Design review of the part built by this model. Coordinates are the model's own, in mm. A direction names the side the tool comes from. Coordinates: 2 decimals unless noted, no trailing zeros. Order: outer loops, then holes, each group sorted by start corner. A loop starts at its lowest first (then second) coordinate and runs counter-clockwise, first axis right, second up. Notation, with made-up numbers: M 71.25,17.25 L 89.25,17.25 A20 ccw 89.25,36.25 Z; hole C 9,-24.5 d10. An arc over 180 degrees is marked long. Answer in a Markdown table with one row per item.
from build123d import *

# Parameters (mm, degrees)
PAD120_DEPTH    = 85
SKETCH241_R     = 1.5
POCKET086_DEPTH = 15.451
SKETCH242_W     = 25
SKETCH242_H     = 15.45
PAD121_DEPTH    = 4


with BuildPart() as part:
    # Sketch240 → Pad120 (new body)
    with BuildSketch(Plane.YZ):
        Polygon((-5.25, 11.45), (-5.25, 15.45), (19.75, 15.45), (19.75, 11.45), (11.25, 11.45), (11.25, 7.15), (14.5, 7.15), (14.5, 0), (0, 0), (0, 7.15), (3.25, 7.15), (3.25, 11.45), align=None)
    extrude(amount=PAD120_DEPTH)

    # Sketch241 (on Face2 of Pad120) → Pocket086 (cut, through all)
    with BuildSketch(Plane(origin=(0, 0, 15.45), x_dir=(0, -1, 0), z_dir=(0, 0, 1))):
        with Locations((-17.25, 77.5)):
            Circle(SKETCH241_R)
        with Locations((-17.25, 52.5)):
            Circle(SKETCH241_R)
        with Locations((2.75, 52.5)):
            Circle(SKETCH241_R)
        with Locations((2.75, 77.5)):
            Circle(SKETCH241_R)
    extrude(amount=-POCKET086_DEPTH, mode=Mode.SUBTRACT)

    # Sketch242 (on Face4 of Pocket086) → Pad121 (join)
    with BuildSketch(Plane(origin=(0, 0, 0), x_dir=(0, 1, 0), z_dir=(-1, 0, 0))):
        with Locations((7.25, -7.725)):
            Rectangle(SKETCH242_W, SKETCH242_H)
    extrude(amount=PAD121_DEPTH)


with BuildPart() as part_1:
    # Body140 placement: moved
    add(part.part.moved(Location((-115, 122.3, 7))))


solid = part_1.part
(1) For faces 4 (the flat face through (-73, 136.8, 11)), 5 (the flat face through (-73, 133.55, 16)), 6 (the cylindrical face through (-37.05, 138.12, 20.48)), 7 (the flat face through (-73, 124, 14.15)), 8 (the flat face through (-73, 122.3, 11)), list the 3-axis set-ups (+Z, -Z, +X, -X, +Y, -Y) from which the entire face can be reached by the end or side of a thin tool; tool diameter is ignored.
Return value:
| item | result |
|---|---|
| face 4 | -Z, +X, +Y |
| face 5 | +X, +Y |
| face 6 | +Z, -Z |
| face 7 | +X, -Y |
| face 8 | -Z, +X, -Y |
(2) Add section C-C, the plane x = -111.5. Give the boundary of the cut face in (y, z).
Return value:
| item | result |
|---|---|
| outline | M 117.05,18.45 L 125.55,18.45 L 125.55,14.15 L 122.3,14.15 L 122.3,7 L 136.8,7 L 136.8,14.15 L 133.55,14.15 L 133.55,18.45 L 142.05,18.45 L 142.05,22.45 L 117.05,22.45 Z |
(3) Add section B-B, the plane y = 139.55. Give the boundary of the cut face in (x, z), and give its area (3 significant figures).
Return value:
| item | result |
|---|---|
| outline | M -119,7 L -115,7 L -115,18.45 L -64,18.45 L -64,22.45 L -119,22.45 Z; M -61,18.45 L -39,18.45 L -39,22.45 L -61,22.45 Z; M -36,18.45 L -30,18.45 L -30,22.45 L -36,22.45 Z |
| area | 378 mm2 |
(4) Insertion check: pin 1 Ø3 at (x, z) = (-99.5, 11.5) entering from +Y; pin 2 Ø1 at (x, y) = (-61.5, 120) entering from -Z; pin 3 Ø1.3 at (x, z) = (-53, 16.5) entering from +Y. Each pin has a flat end and moves straight along its axis. Give the tip position at first contact, or say it passes through.
Return value:
| item | result |
|---|---|
| pin 1 | stops at y = 136.8 |
| pin 2 | stops at z = 18.45 |
| pin 3 | stops at y = 133.55 |
(5) Add section D-D, the plane y = 136. Give the boundary of the cut face in (x, z).
Return value:
| item | result |
|---|---|
| outline | M -119,7 L -30,7 L -30,14.15 L -115,14.15 L -115,18.45 L -30,18.45 L -30,22.45 L -119,22.45 Z |
(6) Draft analysis for pull direction Z (two halves, no side actions). For faces 1 (the cylindrical face through (-38.075, 118.164, 20.478)), 2 (the flat face through (-74, 129, 22.45)), 3 (the flat face through (-73, 135, 14.15)), state which applies: pulls with the +Z half, pulls with the -Z half, needs draft (parallel to the pull), parting line crosses it, or undercut.
Return value:
| item | result |
|---|---|
| face 1 | needs draft |
| face 2 | pulls with the +Z half |
| face 3 | undercut |
(7) For line 1 along Y through (x, z) = (-37.5, 20.55); line 2 along X through (y, z) = (139.5, 20.5); line 3 along Z through (x, y) = (-50, 136.75), list the stretches that pass through material, from the lowest coordinate up. Write a range as from..to.
Return value:
| item | result |
|---|---|
| line 1 | y = 117.05..118.05, 121.05..138.05, 141.05..142.05 |
| line 2 | x = -119..-64, -61..-39, -36..-30 |
| line 3 | z = 7..14.15, 18.45..22.45 |
(8) Add section A-A, the plane x = -37.5. Give the boundary of the cut face in (y, z).
Return value:
| item | result |
|---|---|
| outline | M 117.05,18.45 L 118.05,18.45 L 118.05,22.45 L 117.05,22.45 Z; M 121.05,18.45 L 125.55,18.45 L 125.55,14.15 L 122.3,14.15 L 122.3,7 L 136.8,7 L 136.8,14.15 L 133.55,14.15 L 133.55,18.45 L 138.05,18.45 L 138.05,22.45 L 121.05,22.45 Z; M 141.05,18.45 L 142.05,18.45 L 142.05,22.45 L 141.05,22.45 Z |
